from build123d import *

# Parameters (mm, degrees)
SKETCH1_W           = 100
SKETCH1_H           = 200
SKETCH1_W_2         = 95
SKETCH1_H_2         = 30
BOSS_EXTRUDE1_DEPTH = 5
SKETCH2_R           = 2.1
CUT_EXTRUDE1_DEPTH  = 5
SKETCH3_W           = 20
SKETCH3_H           = 15
SKETCH3_W_2         = 10
SKETCH3_H_2         = 5
BOSS_EXTRUDE2_DEPTH = 5
SKETCH4_R           = 2.1
CUT_EXTRUDE2_DEPTH  = 5
SKETCH5_W           = 30
SKETCH5_H           = 15
SKETCH5_W_2         = 20
SKETCH5_H_2         = 5
BOSS_EXTRUDE3_DEPTH = 5
CUT_EXTRUDE3_DEPTH  = 5
SKETCH7_W           = 5
SKETCH7_H           = 50
CUT_EXTRUDE4_DEPTH  = 5
CUT_EXTRUDE5_DEPTH  = 5
SKETCH9_W           = 5
SKETCH9_H           = 100
CUT_EXTRUDE6_DEPTH  = 5
CUT_EXTRUDE7_DEPTH  = 5


with BuildPart() as part:
    # Sketch1 → Boss-Extrude1 (new body)
    with BuildSketch(Plane.XY):
        Polygon((100, 30), (195, 30), (100, 200), align=None)
        with Locations((50, 100)):
            Rectangle(SKETCH1_W, SKETCH1_H)
        with Locations((147.5, 15)):
            Rectangle(SKETCH1_W_2, SKETCH1_H_2)
    extrude(amount=BOSS_EXTRUDE1_DEPTH)

    # Sketch2 → Cut-Extrude1 (cut)
    with BuildSketch(Plane.XY.offset(5)):
        with Locations((12.1, 6)):
            Circle(SKETCH2_R)
    extrude(amount=-CUT_EXTRUDE1_DEPTH, mode=Mode.SUBTRACT)

    # Sketch3 → Boss-Extrude2 (add)
    # profile 1 of 2: a face of its own
    with BuildSketch(Plane.XY.offset(5)):
        with Locations((20, 207.5)):
            Rectangle(SKETCH3_W, SKETCH3_H)
        with Locations((20, 207.5)):
            Rectangle(SKETCH3_W_2, SKETCH3_H_2, mode=Mode.SUBTRACT)
    # profile 2 of 2: a face of its own
    with BuildSketch(Plane.XY.offset(5)):
        with Locations((80, 207.5)):
            Rectangle(SKETCH3_W, SKETCH3_H)
        with Locations((80, 207.5)):
            Rectangle(SKETCH3_W_2, SKETCH3_H_2, mode=Mode.SUBTRACT)
    extrude(amount=-BOSS_EXTRUDE2_DEPTH)

    # Sketch4 → Cut-Extrude2 (cut)
    with BuildSketch(Plane.XY.offset(5)):
        with Locations((12.1, 11.5)):
            Circle(SKETCH4_R)
        with Locations((12.1, 17)):
            Circle(SKETCH4_R)
    extrude(amount=-CUT_EXTRUDE2_DEPTH, mode=Mode.SUBTRACT)

    # Sketch5 → Boss-Extrude3 (add)
    # profile 1 of 2: a face of its own
    with BuildSketch(Plane.XY.offset(5)):
        with Locations((35, -7.5)):
            Rectangle(SKETCH5_W, SKETCH5_H)
        with Locations((35, -7.5)):
            Rectangle(SKETCH5_W_2, SKETCH5_H_2, mode=Mode.SUBTRACT)
    # profile 2 of 2: a face of its own
    with BuildSketch(Plane.XY.offset(5)):
        with Locations((155, -7.5)):
            Rectangle(SKETCH5_W, SKETCH5_H)
        with Locations((155, -7.5)):
            Rectangle(SKETCH5_W_2, SKETCH5_H_2, mode=Mode.SUBTRACT)
    extrude(amount=-BOSS_EXTRUDE3_DEPTH)

    # Sketch6 → Cut-Extrude3 (cut)
    with BuildSketch(Plane.XY.offset(5)):
        Polygon((100, 169.251038799), (178.051417226, 29.580081657), (174.559643298, 27.628796226), (96.508226071, 167.299753368), align=None)
    extrude(amount=-CUT_EXTRUDE3_DEPTH, mode=Mode.SUBTRACT)

    # Sketch7 → Cut-Extrude4 (cut)
    with BuildSketch(Plane.XY.offset(5)):
        with Locations((72.5, 75)):
            Rectangle(SKETCH7_W, SKETCH7_H)
        with Locations((92.5, 75)):
            Rectangle(SKETCH7_W, SKETCH7_H)
        with Locations((112.5, 75)):
            Rectangle(SKETCH7_W, SKETCH7_H)
    extrude(amount=-CUT_EXTRUDE4_DEPTH, mode=Mode.SUBTRACT)

    # Sketch8 → Cut-Extrude5 (cut)
    with BuildSketch(Plane.XY.offset(5)):
        with BuildLine():
            Line((176.25, 15), (176.25, 5))
            ThreePointArc((176.25, 5), (175, 3.75), (173.75, 5))
            Line((173.75, 5), (173.75, 15))
            ThreePointArc((173.75, 15), (175, 16.25), (176.25, 15))
        make_face()
    extrude(amount=-CUT_EXTRUDE5_DEPTH, mode=Mode.SUBTRACT)

    # Sketch9 → Cut-Extrude6 (cut)
    with BuildSketch(Plane.XY.offset(5)):
        Polygon((78.625722092, 132.677274378), (100.449309145, 144.87280832), (102.888415934, 140.508090909), (81.06482888, 128.312556967), align=None)
        with Locations((12.5, 100)):
            Rectangle(SKETCH9_W, SKETCH9_H)
    extrude(amount=-CUT_EXTRUDE6_DEPTH, mode=Mode.SUBTRACT)

    # Sketch10 → Cut-Extrude7 (cut)
    with BuildSketch(Plane(origin=(0, 0, 0), x_dir=(-1, 0, 0), z_dir=(0, 0, -1))):
        Polygon((-94.582615449, 160.495929169), (-82.387081507, 182.319516222), (-78.022364097, 179.880409434), (-90.217898038, 158.056822381), align=None)
    extrude(amount=-CUT_EXTRUDE7_DEPTH, mode=Mode.SUBTRACT)


solid = part.part
The model under review builds one solid part; all positions refer to its coordinate system, in mm. A direction names the side the tool comes from. Give positions to 0.01 mm unless a question says otherwise; leave off trailing zeros. Order: outer loops, then holes, each group sorted by start corner. A loop starts at its lowest first (then second) coordinate and runs counter-clockwise, first axis right, second up. Notation, with made-up numbers: M 35,-16.5 L 45,-16.5 A34 ccw 45,22.5 Z; hole C -19.5,49 d7. An arc over 180 degrees is marked long. Use one line per item in the form item = value. Start each with the question number.
Item 1: For faces 1 (the flat face through (70, 207, 3)), 2 (the flat face through (15, 207, 3)), 3 (the flat face through (182, 0, 2)), 4 (the flat face through (90, 207, 3)), list the 3-axis set-ups (+Z, -Z, +X, -X, +Y, -Y) from which the entire face can be reached by the end or side of a thin tool; tool diameter is ignored.
Item 2: The part is to be moulded in two halves that separate along X. For faces 5 (the flat face through (155, -5, 3)), 6 (the flat face through (0, 99, 2)), 7 (the flat face through (85, 207, 3)), 8 (the flat face through (80, 215, 3)), say which applies: pulls with the +X half, pulls with the -X half, needs draft (parallel to the pull), parting line crosses it, or undercut.
Item 3: We need section A-A on y = 76.5. Give the boundary of the cut face in (x, z), plus the area to 3 significant figures.
Item 4: We need section C-C on z = 1.65. Give the number of separate pieces and of enclosed holes in the cut face, plus the area to 3 significant figures.
Item 5: We need section B-B on x = 125. Give the boundary of the cut face in (y, z), plus the area to 3 significant figures.
Item 6: Insertion check: pin 1 Ø1.5 at (x, z) = (91.5, 3.5) entering from -Y. The pin has a flat end and moves straight along its axis. Give the tip position at first contact, or say it passes through.
Item 7: We need section D-D on y = 192. Give the boundary of the cut face in (x, z), plus the area to 3 significant figures.
Item 8: To check wall thickness, follow line 1 along Y through (x, z) = (12.1, 2.95); line 2 along Y through (x, z) = (146, 2.1); line 3 along Y through (x, z) = (21, 0.25). State the ranges of each line that lie inside material, in increasing order. Write a range as from..to.
Completed:
q1.face_1 = +Z, -Z, +Y
q1.face_2 = +Z, -Z
q1.face_3 = +Z, -Z, +X, -Y
q1.face_4 = +Z, -Z, +X, +Y
q2.face_5 = undercut
q2.face_6 = pulls with the -X half
q2.face_7 = undercut
q2.face_8 = needs draft
q3.outline = M 0,0 L 10,0 L 10,5 L 0,5 Z; M 15,0 L 70,0 L 70,5 L 15,5 Z; M 75,0 L 90,0 L 90,5 L 75,5 Z; M 95,0 L 110,0 L 110,5 L 95,5 Z; M 115,0 L 147.25,0 L 147.25,5 L 115,5 Z; M 151.83,0 L 169.01,0 L 169.01,5 L 151.83,5 Z
q3.area = 722 mm²
q4.separate_pieces = 1
q4.enclosed_holes = 15
q4.area = 29,900 mm²
q5.outline = M 0,0 L 116.31,0 L 116.31,5 L 0,5 Z; M 124.51,0 L 155.26,0 L 155.26,5 L 124.51,5 Z
q5.area = 735 mm²
q6.pin_1 = 0
q7.outline = M 0,0 L 104.47,0 L 104.47,5 L 0,5 Z
q7.area = 522 mm²
q8.line_1 = 0..3.9, 8.1..9.4, 13.6..14.9, 19.1..50, 150..215
q8.line_2 = -15..-10, -5..78.74, 86.94..117.68
q8.line_3 = -15..205, 210..215
